The listing builds one solid part. Answer for the finished solid, in the listing's coordinates (mm). Round coordinates to 2 decimals unless told otherwise and drop trailing zeros. Write each loop counter-clockwise with the first axis right and the second up, starting at its lowest first coordinate (ties: lowest second). Pieces come first, ordered by that corner, then holes.
Autodesk Inventor part; units mm, degrees
ref_plane "YZ Plane" through (0, 0, 0) normal (1, 0, 0) x (0, 1, 0)
ref_plane "XZ Plane" through (0, 0, 0) normal (0, 1, 0) x (-1, 0, 0)
ref_plane "XY Plane" through (0, 0, 0) normal (0, 0, 1) x (1, 0, 0)
sketch "スケッチ1" plane through (0, 0, 0) normal (0, 0, 1) x (1, 0, 0)
  line L0 (-5.2, -8.25) -> (5.2, -8.25)
  line L1 (5.2, -8.25) -> (5.2, 8.25)
  line L2 (5.2, 8.25) -> (-5.2, 8.25)
  line L3 (-5.2, 8.25) -> (-5.2, -8.25)
  line L4 (-5.2, -8.25) -> (5.2, 8.25) construction
  line L5 (5.2, -8.25) -> (-5.2, 8.25) construction
  point P0 (0, 0)
  dimension "d0" = 10.4
  dimension "d1" = 16.5
extrude "押し出し1" add sketch "スケッチ1" along normal blind 7.6
sketch "スケッチ2" plane through (0, 0, 7.6) normal (0, 0, 1) x (1, 0, 0)
  circle A0 centre (0, -6.95) radius 0.3175
  circle A1 centre (2.5, -6.95) radius 0.3175
  circle A2 centre (-2.5, -6.95) radius 0.3175
  line L0 (-5.2, -8.25) -> (5.2, -8.25)
  point P0 (0, 0)
  dimension "d4" = 1.3
  dimension "d5" = 0.635
  dimension "d6" = 2.5
  dimension "d7" = 2.5
extrude "押し出し2" add sketch "スケッチ2" along normal blind 4.3
properties part number "Circuit_OKI-78SR"
1. Section C-C on z = 8.5 is taken. Give the number of separate pieces and of enclosed holes in the cut face, plus the area to 3 significant figures.
Geometry says:
separate pieces: 3
enclosed holes: 0
area: 0.950 mm2
2. Section B-B on x = 2.5 is taken. Determine the outline of the cut face in (y, z).
Geometry says:
outline: (-8.25, 0) - (8.25, 0) - (8.25, 7.6) - (-6.63, 7.6) - (-6.63, 11.9) - (-7.27, 11.9) - (-7.27, 7.6) - (-8.25, 7.6) - close
3. Section A-A on y = -6.95 is taken. Determine the outline of the cut face in (x, z), plus the area to 3 significant figures.
Geometry says:
outline: (-5.2, 0) - (5.2, 0) - (5.2, 7.6) - (2.82, 7.6) - (2.82, 11.9) - (2.18, 11.9) - (2.18, 7.6) - (0.32, 7.6) - (0.32, 11.9) - (-0.32, 11.9) - (-0.32, 7.6) - (-2.18, 7.6) - (-2.18, 11.9) - (-2.82, 11.9) - (-2.82, 7.6) - (-5.2, 7.6) - close
area: 87.2 mm2
4. Given pin 1 (4 mm diameter, centred on x = -0.5, y = -3, fed in from +Z), flat-ended and moving along its own axis, determine where the tip first touches the part or whether it passes through.
Geometry says:
pin 1: stops at z = 7.6
5. Section D-D on y = 4.75 is taken. Determine the outline of the cut face in (x, z).
Geometry says:
outline: (-5.2, 0) - (5.2, 0) - (5.2, 7.6) - (-5.2, 7.6) - close
6. Straight lines are drawn through the part: line 1 along X through (y, z) = (-7, 10.5); line 2 along Z through (x, y) = (4.5, 0.5); line 3 along Y through (x, z) = (-2.5, 8.75). For each, find the intervals that lie inside material, in ascending order.
Geometry says:
line 1: x = -2.81 to -2.19, -0.31 to 0.31, 2.19 to 2.81
line 2: z = 0 to 7.6
line 3: y = -7.27 to -6.63
